The model under review builds one solid part; all positions refer to its coordinate system, in mm. A direction names the side the tool comes from. Round coordinates to 2 decimals unless told otherwise and drop trailing zeros. Order: outer loops, then holes, each group sorted by start corner. A loop starts at its lowest first (then second) coordinate and runs counter-clockwise, first axis right, second up. Notation, with made-up numbers: (74.5, -8.5) - (98.5, -8.5) arc R32 cw to (98.5, 26.5) - close; hole circle Ø6 at (45, 34). An arc over 180 degrees is marked (long way). One line per question, with ' | ' between items. Start each with the question number.
Item 1: Add section C-C on y = -3.75. State the section outline as (x, z) points (3 decimals), and give its area (3 significant figures).
Item 2: Add section D-D on x = -7. State the section outline as (y, z) points, and give its area (3 significant figures).
Item 3: Add section A-A on x = 12.5. State the section outline as (y, z) points.
Item 4: Insertion check: pin 1 Ø1.5 at (x, z) = (9.5, 10) entering from -Y; pin 2 Ø8 at (x, z) = (11.5, 6) entering from +Y; pin 3 Ø5 at (x, z) = (-7.5, 5) entering from -Y. Each pin has a flat end and moves straight along its axis. Give the tip position at first contact, or say it passes through.
Item 5: For L1, parallel to Y at x = 6, z = 6.5; L2, parallel to Y at x = 13.5, z = 14, list the stretches that pass through material, from the lowest coordinate up. Write a range as [from, to].
Item 6: Tool access review of faces 5 (the face through (11, 6.65, 8)), 6 (the face through (-9, 1.013, 8)), 7 (the face through (10, 0, 14.716)), 8 (the face through (11, -6.65, 8)): name each direction out of +Z, -Z, +X, -X, +Y, -Y from which nothing blocks a thin tool from reaching the whole face with its end or side.
Item 7: Add section B-B on z = 6. State the section outline as (x, y) points (3 decimals), and give its area (3 significant figures).
Item 8: Draft analysis for pull direction Y (two halves, no side actions). For faces 1 (the face through (3.166, -7.598, 8.12)), 2 (the face through (9, 0, 13.216)), 3 (the face through (2.9, 0.11, 15.06)), 4 (the face through (9, -5.15, 8)), state which applies: +Y half, -Y half, draft (parallel to the pull), parting line (faces both ways), or undercut.
from build123d import *

# Parameters (mm, degrees)
F0_W         = 2.75
F0_H         = 20
F1_DEPTH     = 16
F2_W         = 5.15
F2_H         = 10.3
F3_DEPTH     = 2.75
F4_DEPTH     = 15
F5_T1_DEPTH  = 13.2999992773
F5_T3_DEPTH  = 13.2999992773
F5_T9_DEPTH  = 21.6634917276
F5_T14_DEPTH = 25.0997612432
F5_T22_DEPTH = 21.6634917276
F5_T27_DEPTH = 25.0997612432
F5_T35_DEPTH = 22.0158699277
F5_T40_DEPTH = 25.0997612432
F5_T48_DEPTH = 25.0997612432
F5_T53_DEPTH = 22.0158699277
F6_R         = 5
F7_W         = 2
F7_H         = 16
F8_DEPTH     = 16


# Not quite as in the source:
# - a fillet or chamfer that OpenCascade refuses, or shapes differently, is made with other operations: its cross-section is extruded or revolved along the edge and cut away or added
# - a feature names something its author has since deleted; it is built from what else it names


with BuildPart() as f1:
    # F0 (on Top) → F1 (new body)
    with BuildSketch(Plane.XY):
        Rectangle(F0_W, F0_H)
    extrude(amount=F1_DEPTH)

    # F2 (on face) → F3 (join)
    with BuildSketch(Plane.YZ.offset(1.375)):
        Polygon((0, 16), (-10, 16), (-10, 0), (0, 0), (0, 1.4159553841), (-6.6499996386, 1.4159553841), (-6.6499996386, 14.7159546614), (0, 14.7159546614), align=None)
        Polygon((10, 16), (0, 16), (0, 14.7159546614), (6.6499996386, 14.7159546614), (6.6499996386, 1.4159553841), (0, 1.4159553841), (0, 0), (10, 0), align=None)
        with Locations((-2.575, 8.0659550227)):
            Rectangle(F2_W, F2_H)
        with Locations((2.575, 8.0659550227)):
            Rectangle(F2_W, F2_H)
        Polygon((0, 13.2159550227), (0, 14.7159546614), (-6.6499996386, 14.7159546614), (-6.6499996386, 1.4159553841), (0, 1.4159553841), (0, 2.9159550227), (-5.15, 2.9159550227), (-5.15, 13.2159550227), align=None)
        Polygon((6.6499996386, 14.7159546614), (0, 14.7159546614), (0, 13.2159550227), (5.15, 13.2159550227), (5.15, 2.9159550227), (0, 2.9159550227), (0, 1.4159553841), (6.6499996386, 1.4159553841), align=None)
    extrude(amount=-F3_DEPTH)

    # F2 (on face) → F4 (join)
    with BuildSketch(Plane.YZ.offset(1.375)):
        Polygon((0, 13.2159550227), (0, 14.7159546614), (-6.6499996386, 14.7159546614), (-6.6499996386, 1.4159553841), (0, 1.4159553841), (0, 2.9159550227), (-5.15, 2.9159550227), (-5.15, 13.2159550227), align=None)
        Polygon((6.6499996386, 14.7159546614), (0, 14.7159546614), (0, 13.2159550227), (5.15, 13.2159550227), (5.15, 2.9159550227), (0, 2.9159550227), (0, 1.4159553841), (6.6499996386, 1.4159553841), align=None)
    extrude(amount=F4_DEPTH)

    # F5: fillet of radius 5 on 6 edges, made by hand

    # F5_s2 → F5_t1 (join)
    with BuildSketch(Plane.XZ.offset(-6.6499996386)):
        with BuildLine():
            ThreePointArc((1.375, 16), (2.9287180617, 15.0479907955), (4.7203969801, 14.7159546614))
            Line((4.7203969801, 14.7159546614), (1.375, 14.7159546614))
            Line((1.375, 14.7159546614), (1.375, 16))
        make_face()
        with BuildLine():
            ThreePointArc((1.375, 0), (2.9798891295, 1.0484613517), (4.8613482602, 1.4159553841))
            Line((4.8613482602, 1.4159553841), (1.375, 1.4159553841))
            Line((1.375, 1.4159553841), (1.375, 0))
        make_face()
    extrude(amount=F5_T1_DEPTH)

    # F5_s4 → F5_t3 (join)
    with BuildSketch(Plane.XY.offset(1.4159553841)):
        with BuildLine():
            ThreePointArc((1.375, -10), (3.2009454046, -7.5726231419), (6.0949047864, -6.6499996386))
            Line((6.0949047864, -6.6499996386), (1.375, -6.6499996386))
            Line((1.375, -6.6499996386), (1.375, -10))
        make_face()
        with BuildLine():
            ThreePointArc((1.375, 10), (3.2009454046, 7.5726231419), (6.0949047864, 6.6499996386))
            Line((6.0949047864, 6.6499996386), (1.375, 6.6499996386))
            Line((1.375, 6.6499996386), (1.375, 10))
        make_face()
    extrude(amount=F5_T3_DEPTH)


with BuildPart() as f5_tool7:
    # F5_s8 → F5_t9 (new body)
    with BuildSketch(Plane.XZ.offset(-15.013492089)):
        with BuildLine():
            ThreePointArc((1.375, 16), (2.9287180617, 15.0479907955), (4.7203969801, 14.7159546614))
            Line((4.7203969801, 14.7159546614), (1.375, 14.7159546614))
            Line((1.375, 14.7159546614), (1.375, 16))
        make_face()
    extrude(amount=F5_T9_DEPTH)

    split(bisect_by=Plane.XZ.offset(-10), keep=Keep.TOP)

    split(bisect_by=Plane.XZ.offset(-6.6499996386), keep=Keep.BOTTOM)


with BuildPart() as f5_tool12:
    # F5_s13 → F5_t14 (new body)
    with BuildSketch(Plane.XY.offset(1.4159553841)):
        with BuildLine():
            ThreePointArc((1.375, 10), (3.2009454046, 7.5726231419), (6.0949047864, 6.6499996386))
            Line((6.0949047864, 6.6499996386), (1.375, 6.6499996386))
            Line((1.375, 6.6499996386), (1.375, 10))
        make_face()
    extrude(amount=F5_T14_DEPTH)

    split(bisect_by=Plane.XY.offset(16), keep=Keep.BOTTOM)

    split(bisect_by=Plane.XY.offset(14.7159546614), keep=Keep.TOP)


with BuildPart() as f5_tool7_1:
    add(f5_tool7.part)

    # F5_t17: intersect F5_tool12
    add(f5_tool12.part, mode=Mode.INTERSECT)


with BuildPart() as f1_1:
    add(f1.part)

    # F5_t5: union F5_tool7
    add(f5_tool7_1.part)


with BuildPart() as f5_tool20:
    # F5_s21 → F5_t22 (new body)
    with BuildSketch(Plane.XZ.offset(-6.6499996386)):
        with BuildLine():
            ThreePointArc((1.375, 16), (2.9287180617, 15.0479907955), (4.7203969801, 14.7159546614))
            Line((4.7203969801, 14.7159546614), (1.375, 14.7159546614))
            Line((1.375, 14.7159546614), (1.375, 16))
        make_face()
    extrude(amount=F5_T22_DEPTH)

    split(bisect_by=Plane.XZ.offset(10), keep=Keep.BOTTOM)

    split(bisect_by=Plane.XZ.offset(6.6499996386), keep=Keep.TOP)


with BuildPart() as f5_tool25:
    # F5_s26 → F5_t27 (new body)
    with BuildSketch(Plane.XY.offset(26.5157166273)):
        with BuildLine():
            ThreePointArc((1.375, -10), (3.2009454046, -7.5726231419), (6.0949047864, -6.6499996386))
            Line((6.0949047864, -6.6499996386), (1.375, -6.6499996386))
            Line((1.375, -6.6499996386), (1.375, -10))
        make_face()
    extrude(amount=-F5_T27_DEPTH)

    split(bisect_by=Plane.XY.offset(16), keep=Keep.BOTTOM)

    split(bisect_by=Plane.XY.offset(14.7159546614), keep=Keep.TOP)


with BuildPart() as f5_tool20_1:
    add(f5_tool20.part)

    # F5_t30: intersect F5_tool25
    add(f5_tool25.part, mode=Mode.INTERSECT)


with BuildPart() as f1_2:
    add(f1_1.part)

    # F5_t18: union F5_tool20
    add(f5_tool20_1.part)


with BuildPart() as f5_tool33:
    # F5_s34 → F5_t35 (new body)
    with BuildSketch(Plane.XZ.offset(15.365870289)):
        with BuildLine():
            ThreePointArc((1.375, 0), (2.9798891295, 1.0484613517), (4.8613482602, 1.4159553841))
            Line((4.8613482602, 1.4159553841), (1.375, 1.4159553841))
            Line((1.375, 1.4159553841), (1.375, 0))
        make_face()
    extrude(amount=-F5_T35_DEPTH)

    split(bisect_by=Plane.XZ.offset(10), keep=Keep.BOTTOM)

    split(bisect_by=Plane.XZ.offset(6.6499996386), keep=Keep.TOP)


with BuildPart() as f5_tool38:
    # F5_s39 → F5_t40 (new body)
    with BuildSketch(Plane.XY.offset(14.7159546614)):
        with BuildLine():
            ThreePointArc((1.375, -10), (3.2009454046, -7.5726231419), (6.0949047864, -6.6499996386))
            Line((6.0949047864, -6.6499996386), (1.375, -6.6499996386))
            Line((1.375, -6.6499996386), (1.375, -10))
        make_face()
    extrude(amount=-F5_T40_DEPTH)

    split(bisect_by=Plane.XY, keep=Keep.TOP)

    split(bisect_by=Plane.XY.offset(1.4159553841), keep=Keep.BOTTOM)


with BuildPart() as f5_tool33_1:
    add(f5_tool33.part)

    # F5_t43: intersect F5_tool38
    add(f5_tool38.part, mode=Mode.INTERSECT)


with BuildPart() as f1_3:
    add(f1_2.part)

    # F5_t31: union F5_tool33
    add(f5_tool33_1.part)


with BuildPart() as f5_tool46:
    # F5_s47 → F5_t48 (new body)
    with BuildSketch(Plane.XY.offset(-10.3838065819)):
        with BuildLine():
            ThreePointArc((1.375, 10), (3.2009454046, 7.5726231419), (6.0949047864, 6.6499996386))
            Line((6.0949047864, 6.6499996386), (1.375, 6.6499996386))
            Line((1.375, 6.6499996386), (1.375, 10))
        make_face()
    extrude(amount=F5_T48_DEPTH)

    split(bisect_by=Plane.XY, keep=Keep.TOP)

    split(bisect_by=Plane.XY.offset(1.4159553841), keep=Keep.BOTTOM)


with BuildPart() as f5_tool51:
    # F5_s52 → F5_t53 (new body)
    with BuildSketch(Plane.XZ.offset(6.6499996386)):
        with BuildLine():
            ThreePointArc((1.375, 0), (2.9798891295, 1.0484613517), (4.8613482602, 1.4159553841))
            Line((4.8613482602, 1.4159553841), (1.375, 1.4159553841))
            Line((1.375, 1.4159553841), (1.375, 0))
        make_face()
    extrude(amount=-F5_T53_DEPTH)

    split(bisect_by=Plane.XZ.offset(-10), keep=Keep.TOP)

    split(bisect_by=Plane.XZ.offset(-6.6499996386), keep=Keep.BOTTOM)


with BuildPart() as f5_tool46_1:
    add(f5_tool46.part)

    # F5_t56: intersect F5_tool51
    add(f5_tool51.part, mode=Mode.INTERSECT)


with BuildPart() as f1_4:
    add(f1_3.part)

    # F5_t44: union F5_tool46
    add(f5_tool46_1.part)

    # F6
    f6_edges = [f1_4.edges().sort_by_distance(p)[0] for p in [
        (0, -10, 0),
        (0, -10, 16),
        (0, 10, 16),
        (0, 10, 0),
    ]]
    fillet(f6_edges, radius=F6_R)

    # F7 (on face) → F8 (join)
    with BuildSketch(Plane(origin=(-1.375, 0, 0), x_dir=(0, -1, 0), z_dir=(-1, 0, 0))):
        with Locations((-0.0132987518, 8)):
            Rectangle(F7_W, F7_H)
    extrude(amount=F8_DEPTH)


solid = f1_4.part
Determined:
1) outline: (-1.375, 0) - (1.375, 0) arc R5 cw to (4.861, 1.416) - (16.375, 1.416) - (16.375, 2.916) - (1.375, 2.916) - (1.375, 13.216) - (16.375, 13.216) - (16.375, 14.716) - (4.72, 14.716) arc R5 cw to (1.375, 16) - (-1.375, 16) - close | area: 91.9 mm2
2) outline: (-0.99, 0) - (1.01, 0) - (1.01, 16) - (-0.99, 16) - close | area: 32.0 mm2
3) outline: (-6.65, 1.42) - (6.65, 1.42) - (6.65, 14.72) - (-6.65, 14.72) - close; hole (-5.15, 2.92) - (5.15, 2.92) - (5.15, 13.22) - (-5.15, 13.22) - close
4) pin 1: y = -6.65 | pin 2: y = 6.65 | pin 3: y = -0.99
5) L1: [-6.65, -5.15], [5.15, 6.65] | L2: [-6.65, 6.65]
6) face 5: +Z, -Z, +X, +Y | face 6: +Z, -Z, -X, +Y | face 7: +Z, +X, +Y, -Y | face 8: +Z, -Z, +X, -Y
7) outline: (-17.375, -0.987) - (-1.375, -0.987) - (-1.375, -10) - (1.375, -10) arc R5 cw to (6.095, -6.65) - (16.375, -6.65) - (16.375, -5.15) - (1.375, -5.15) - (1.375, 5.15) - (16.375, 5.15) - (16.375, 6.65) - (6.095, 6.65) arc R5 cw to (1.375, 10) - (-1.375, 10) - (-1.375, 1.013) - (-17.375, 1.013) - close | area: 141 mm2
8) face 1: -Y half | face 2: undercut | face 3: draft | face 4: undercut
